```python
from build123d import *

# Parameters (mm, degrees)
BOSS_EXTRUDE1_DEPTH     = 7.5
BOSS_EXTRUDE2_DEPTH     = 60
SCALE1_SCALE            = 0.27
FILLET1_R               = 3
CUT_EXTRUDE1_DEPTH      = 33.359704853
CUT_EXTRUDE1_DEPTH_BACK = 33.359704853
SKETCH3_R               = 1.5


with BuildPart() as part:
    # Sketch1 → Boss-Extrude1 (new body)
    with BuildSketch(Plane(origin=(0, 0, 0), x_dir=(1, 0, 0), z_dir=(0, 1, 0))):
        with BuildLine():
            Line((-59.846085345, 60.187558837), (-43, -67.771163202))
            Line((-43, -67.771163202), (43, -67.771163202))
            Line((43, -67.771163202), (59.846085345, 60.187558837))
            ThreePointArc((59.846085345, 60.187558837), (0, 66), (-59.846085345, 60.187558837))
        make_face()
    boss_extrude1 = extrude(amount=BOSS_EXTRUDE1_DEPTH)

    # Sketch2 → Boss-Extrude2 (add)
    with BuildSketch(Plane(origin=(0, 7.5, 0), x_dir=(1, 0, 0), z_dir=(0, 1, 0))):
        with BuildLine():
            Line((16.954011105, -35.771163202), (26.24120117, 34.772048928))
            ThreePointArc((26.24120117, 34.772048928), (0, 36), (-26.24120117, 34.772048928))
            Line((-26.24120117, 34.772048928), (-16.954011105, -35.771163202))
            Line((-16.954011105, -35.771163202), (16.954011105, -35.771163202))
        make_face()
    extrude(amount=BOSS_EXTRUDE2_DEPTH)

    # Mirror1: Boss-Extrude1 across plane
    add(boss_extrude1.mirror(Plane.ZX.offset(37.5)))


with BuildPart() as part_1:
    # Scale1: scaled about (0, 37.5, -2.151413181)
    add(part.part.scale(SCALE1_SCALE).moved(Location((0, 27.375, -1.570531622))))

    # Fillet1
    fillet1_edges = [part_1.edges().sort_by_distance(p)[0] for p in [
        (4.577582998, 37.5, 8.087682442),
        (7.085124316, 37.5, -10.958984833),
        (-7.085124316, 37.5, -10.958984833),
        (-4.577582998, 37.5, 8.087682442),
    ]]
    fillet(fillet1_edges, radius=FILLET1_R)

    # Sketch3 → Cut-Extrude1 (cut, two sides: drawn at the far end of the back side and taken through both)
    with BuildSketch(Plane(origin=(0, 47.625, 0), x_dir=(1, 0, 0), z_dir=(0, 1, 0)).offset(-CUT_EXTRUDE1_DEPTH_BACK)):
        with BuildLine():
            ThreePointArc((3.239363531, -3.696003073), (2.492140677, -5.093958707), (1.008612593, -5.65231697))
            Line((1.008612593, -5.65231697), (-1.008612593, -5.65231697))
            ThreePointArc((-1.008612593, -5.65231697), (-2.492140855, -5.093956631), (-3.239363817, -3.696000902))
            Line((-3.239363817, -3.696000902), (-4.667928785, 7.155027331))
            ThreePointArc((-4.667928785, 7.155027331), (-4.128817414, 8.932239348), (-2.437177847, 9.698711264))
            Line((-2.437177847, 9.698711264), (2.437177847, 9.698711264))
            ThreePointArc((2.437177847, 9.698711264), (4.128817414, 8.932239348), (4.667928785, 7.155027331))
            Line((4.667928785, 7.155027331), (3.239363531, -3.696003073))
        make_face()
        with Locations(Location((2.5, 16.890531622, 0), (0, 0, 270))):
            Circle(SKETCH3_R)
        with Locations(Location((-2.5, 16.890531622, 0), (0, 0, 270))):
            Circle(SKETCH3_R)
        with Locations(Location((-2.5, -14.227682443, 0), (0, 0, 270))):
            Circle(SKETCH3_R)
        with Locations(Location((2.5, -14.227682443, 0), (0, 0, 270))):
            Circle(SKETCH3_R)
    extrude(amount=CUT_EXTRUDE1_DEPTH + CUT_EXTRUDE1_DEPTH_BACK, mode=Mode.SUBTRACT)


solid = part_1.part
```
Geometry: final body of the model. Coordinates: model frame, mm. A direction names the side the tool comes from. Round coordinates to 2 decimals unless told otherwise and drop trailing zeros. Loops run counter-clockwise (first coordinate to the right, second up) from the corner with the lowest first, then second, coordinate; pieces in that order, holes last. Notation, with made-up numbers: (33.25, 30) -> (54.25, 30) arc R17 ccw to (54.25, 47) -> close; hole circle Ø6 at (7.25, 9.25). An arc over 180 degrees is marked (long way). Write each question's results on one line, items separated by ' | '.
Item 1: Pull-direction query (Y, two-part tool) for faces 6 (the face through (6.023, 37.613, -10.09)), 7 (the face through (3.964, 37.358, -1.805)), 8 (the face through (-4, 47.625, 2)); classes: pulls with the +Y half, pulls with the -Y half, needs draft (parallel to the pull), parting line crosses it, or undercut.
Answers below:
face 6: undercut | face 7: needs draft | face 8: pulls with the +Y half
Item 2: Cut plane C-C on z = 9.5. Return the cut outline in (x, y) (3 decimals).
Answers below:
outline: (-12.562, 27.375) -> (12.562, 27.375) -> (12.562, 29.4) -> (-12.562, 29.4) -> close; (-12.562, 45.6) -> (12.562, 45.6) -> (12.562, 47.625) -> (-12.562, 47.625) -> close
Item 3: Cut plane A-A on y = 33. Return the cut outline in (x, z).
Answers below:
outline: (-6.67, -7.81) arc R3 ccw to (-3.85, -11.19) arc R75.87 ccw to (3.85, -11.19) arc R3 ccw to (6.67, -7.81) -> (4.92, 5.48) arc R3 ccw to (1.95, 8.09) -> (-1.95, 8.09) arc R3 ccw to (-4.92, 5.48) -> close; hole (-4.67, -7.16) arc R2.25 ccw to (-2.44, -9.7) -> (2.44, -9.7) arc R2.25 ccw to (4.67, -7.16) -> (3.24, 3.7) arc R2.25 ccw to (1.01, 5.65) -> (-1.01, 5.65) arc R2.25 ccw to (-3.24, 3.7) -> close
Item 4: Set-up query: faces 1 (the face through (-4.15, 37.36, -8.91)), 2 (the face through (3.95, 37.61, 7.32)), 3 (the face through (13.85, 28.37, -0.3)), 4 (the face through (0.05, 37.39, -11.29)), 5 (the face through (-3.95, 37.61, 7.32)). Return all of +Z, -Z, +X, -X, +Y, -Y with unobstructed straight access to the full face (end or side cutting, diameter ignored); none if empty.
Answers below:
face 1: +Y, -Y | face 2: +Z, +X | face 3: +Z, +X, +Y, -Y | face 4: -Z | face 5: +Z, -X
Item 5: Cut plane B-B on x = 7.5. Return the cut outline in (y, z) (3 decimals).
Answers below:
outline: (27.375, -19.055) -> (29.4, -19.055) -> (29.4, 16.728) -> (27.375, 16.728) -> close; (45.6, -19.055) -> (47.625, -19.055) -> (47.625, 16.728) -> (45.6, 16.728) -> close
Item 6: Cut plane D-D on y = 46.5. Return the cut outline in (x, z).
Answers below:
outline: (-16.16, -17.82) arc R83.97 ccw to (16.16, -17.82) -> (11.61, 16.73) -> (-11.61, 16.73) -> close; hole (-4.67, -7.16) arc R2.25 ccw to (-2.44, -9.7) -> (2.44, -9.7) arc R2.25 ccw to (4.67, -7.16) -> (3.24, 3.7) arc R2.25 ccw to (1.01, 5.65) -> (-1.01, 5.65) arc R2.25 ccw to (-3.24, 3.7) -> close; hole circle Ø3 at (-2.5, -16.89); hole circle Ø3 at (-2.5, 14.23); hole circle Ø3 at (2.5, -16.89); hole circle Ø3 at (2.5, 14.23)
Item 7: Pin query (flat end, axial travel): pin 1 Ø12 at (y, z) = (36.5, -3) entering from -X; pin 2 Ø2 at (x, y) = (0.5, 33) entering from -Z; pin 3 Ø4.5 at (x, y) = (0, 38.5) entering from +Z; pin 4 Ø1.8 at (x, z) = (2.5, 14.23) entering from +Y. Return the tip coordinate at first contact, or that it passes through.
Answers below:
pin 1: stops at x = -6.7 | pin 2: stops at z = -11.29 | pin 3: stops at z = 8.09 | pin 4: passes through
Item 8: Line query: probe 1 along Y at (x, z) = (-9.5, -14) (3 decimals); probe 2 along Z at (x, y) = (-2.5, 28.25); probe 3 along X at (y, z) = (46, 7). Output: solid intervals per line, ascending. Write a range as [from, to].
Answers below:
probe 1: y = [27.375, 29.4], [45.6, 47.625] | probe 2: z = [-19.35, -18.39], [-15.39, -9.7], [5.09, 12.73], [15.73, 16.73] | probe 3: x = [-12.89, 12.89]
